Answer from the drawing. Dimensions are ordinates in mm from the lowest x, y and z of the part. Coordinates: 2 decimals unless noted, no trailing zeros. Write each loop counter-clockwise with the first axis right and the second up, starting at its lowest first coordinate (ties: lowest second). Pieces come first, ordered by that corner, then holes. Notation, with made-up numbers: (59, -24.75) -> (68, -24.75) arc R20 ccw to (68, 12.25) -> close; hole circle Ø2 at (37.5, 57.25). An arc over 180 degrees is marked (long way). One line per item, written item: value. Start each with the question number.
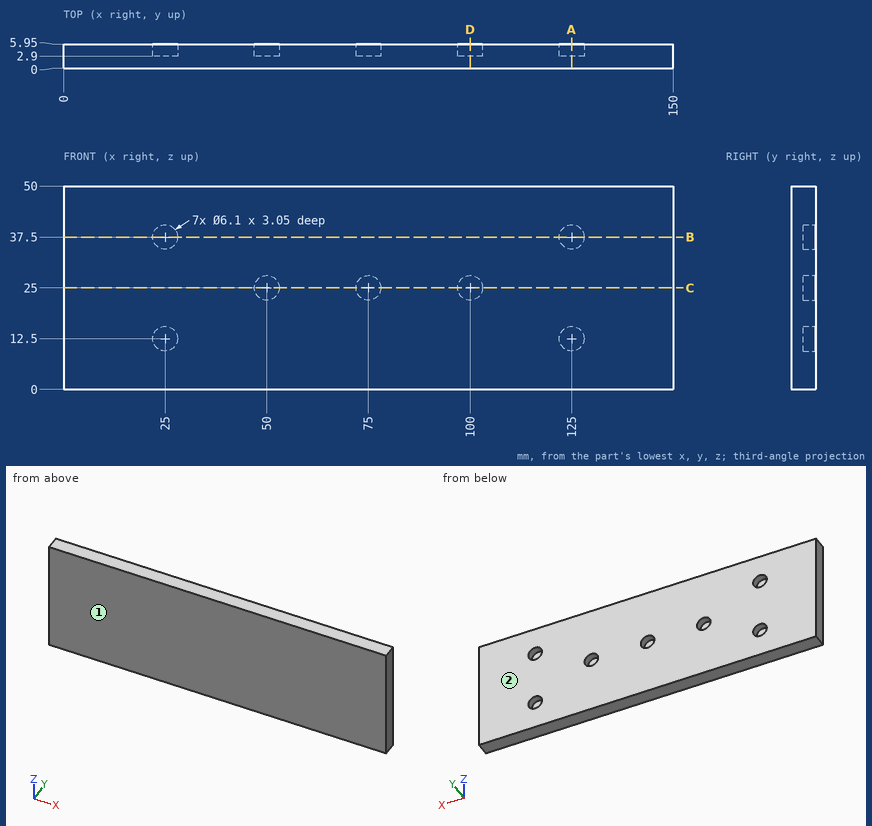
1. A cutting plane is placed at C-C on z = 25. Give the vertices of the cut face in (x, y), then the cut area to 3 significant figures.
2. Find the intervals of material crossed by probe 1 along X at (y, z) = (5.3, 25); probe 2 along X at (y, z) = (5, 12.5); probe 3 along Z at (x, y) = (125, 5.1), in increasing order. Write a range as from..to.
3. A cutting plane is placed at B-B on z = 37.5. Give the vertices of the cut face in (x, y).
4. A cutting plane is placed at A-A on x = 125. Give the vertices of the cut face in (y, z).
5. Given pin 1 (3 mm diameter, centred on x = 126, z = 37.5, fed in from +Y), flat-ended and moving along its own axis, determine where the tip first touches the part or whether it passes through.
6. For a pull along Y with two mould halves and no side action, classify the marked faces 1 and 2 as +Y half, -Y half, draft (parallel to the pull), parting line (faces both ways), or undercut.
7. A cutting plane is placed at D-D on x = 100. Give the vertices of the cut face in (y, z), then the cut area to 3 significant figures.
Derived:
1. outline: (0, 0) -> (150, 0) -> (150, 5.95) -> (103.05, 5.95) -> (103.05, 2.9) -> (96.95, 2.9) -> (96.95, 5.95) -> (78.05, 5.95) -> (78.05, 2.9) -> (71.95, 2.9) -> (71.95, 5.95) -> (53.05, 5.95) -> (53.05, 2.9) -> (46.95, 2.9) -> (46.95, 5.95) -> (0, 5.95) -> close
1. area: 837 mm2
2. probe 1: x = 0..46.95, 53.05..71.95, 78.05..96.95, 103.05..150
2. probe 2: x = 0..21.95, 28.05..121.95, 128.05..150
2. probe 3: z = 0..9.45, 15.55..34.45, 40.55..50
3. outline: (0, 0) -> (150, 0) -> (150, 5.95) -> (128.05, 5.95) -> (128.05, 2.9) -> (121.95, 2.9) -> (121.95, 5.95) -> (28.05, 5.95) -> (28.05, 2.9) -> (21.95, 2.9) -> (21.95, 5.95) -> (0, 5.95) -> close
4. outline: (0, 0) -> (5.95, 0) -> (5.95, 9.45) -> (2.9, 9.45) -> (2.9, 15.55) -> (5.95, 15.55) -> (5.95, 34.45) -> (2.9, 34.45) -> (2.9, 40.55) -> (5.95, 40.55) -> (5.95, 50) -> (0, 50) -> close
5. pin 1: stops at y = 2.9
6. face 1: -Y half
6. face 2: +Y half
7. outline: (0, 0) -> (5.95, 0) -> (5.95, 21.95) -> (2.9, 21.95) -> (2.9, 28.05) -> (5.95, 28.05) -> (5.95, 50) -> (0, 50) -> close
7. area: 279 mm2
